Source: CAD feature listing. Evaluate the final solid. Frame: model axes, mm. Round coordinates to 2 decimals unless told otherwise and drop trailing zeros. Use one line per item in the form item = value. Start each with the question number.
Q1. Ray query, line 1 (X direction, y = 5.25, z = 22.5); line 2 (Z direction, x = -54, y = 3.25) (3 decimals). Return the intervals inside material, ascending. Write a range as [from, to].
Q2. Pin query (flat end, axial travel): pin 1 Ø4 at (x, z) = (-88, 31) entering from -Y; pin 2 Ø3 at (x, y) = (169.5, 4.5) entering from +Z (3 decimals). Return the tip coordinate at first contact, or that it passes through.
Q3. Cut plane A-A, the plane z = 34. Give the number of separate pieces and of enclosed holes in the cut face, and give its area (3 significant figures).
from build123d import *

# Parameters (mm, degrees)
SKETCH1_W           = 647.7
SKETCH1_H           = 57.15
BOSS_EXTRUDE1_DEPTH = 6.35
SKETCH3_W           = 24.892
SKETCH3_H           = 12
BOSS_EXTRUDE2_DEPTH = 6.35
SKETCH4_W           = 13.208
SKETCH4_H           = 13.208
CUT_EXTRUDE2_DEPTH  = 327.443679101
SKETCH5_W           = 647.7
SKETCH5_H           = 6.35
CUT_EXTRUDE3_DEPTH  = 31.304


with BuildPart() as part:
    # Sketch1 → Boss-Extrude1 (new body)
    with BuildSketch(Plane(origin=(0, 0, 0), x_dir=(1, 0, 0), z_dir=(0, 1, 0))):
        Rectangle(SKETCH1_W, SKETCH1_H)
    extrude(amount=BOSS_EXTRUDE1_DEPTH)

    # Sketch3 → Boss-Extrude2 (add)
    with BuildSketch(Plane(origin=(0, 0, 0), x_dir=(1, 0, 0), z_dir=(0, 1, 0))):
        Polygon((-317.5, -40.575), (-292.608, -40.575), (-292.608, -28.575), (-317.5, -28.575), (-323.85, -28.575), (-323.85, -40.575), align=None)
        with Locations((-266.954, -34.575)):
            Rectangle(SKETCH3_W, SKETCH3_H)
        with Locations((-228.854, -34.575)):
            Rectangle(SKETCH3_W, SKETCH3_H)
        with Locations((-190.754, -34.575)):
            Rectangle(SKETCH3_W, SKETCH3_H)
        with Locations((-152.654, -34.575)):
            Rectangle(SKETCH3_W, SKETCH3_H)
        with Locations((-114.554, -34.575)):
            Rectangle(SKETCH3_W, SKETCH3_H)
        with Locations((-76.454, -34.575)):
            Rectangle(SKETCH3_W, SKETCH3_H)
        with Locations((-38.354, -34.575)):
            Rectangle(SKETCH3_W, SKETCH3_H)
        with Locations((-0.254, -34.575)):
            Rectangle(SKETCH3_W, SKETCH3_H)
        with Locations((37.846, -34.575)):
            Rectangle(SKETCH3_W, SKETCH3_H)
        with Locations((75.946, -34.575)):
            Rectangle(SKETCH3_W, SKETCH3_H)
        with Locations((114.046, -34.575)):
            Rectangle(SKETCH3_W, SKETCH3_H)
        with Locations((152.146, -34.575)):
            Rectangle(SKETCH3_W, SKETCH3_H)
        with Locations((190.246, -34.575)):
            Rectangle(SKETCH3_W, SKETCH3_H)
        with Locations((228.346, -34.575)):
            Rectangle(SKETCH3_W, SKETCH3_H)
        with Locations((266.446, -34.575)):
            Rectangle(SKETCH3_W, SKETCH3_H)
        Polygon((316.992, -28.575), (292.1, -28.575), (292.1, -40.575), (316.992, -40.575), (323.85, -40.575), (323.85, -28.575), align=None)
    extrude(amount=BOSS_EXTRUDE2_DEPTH)

    # Sketch4 → Cut-Extrude2 (cut, through all)
    with BuildSketch(Plane(origin=(0, 0, 0), x_dir=(1, 0, 0), z_dir=(0, 1, 0))):
        with Locations((-323.85, 3.875)):
            Rectangle(SKETCH4_W, SKETCH4_H)
        with Locations((-323.85, -22.133)):
            Rectangle(SKETCH4_W, SKETCH4_H)
        with Locations((323.85, -22.133)):
            Rectangle(SKETCH4_W, SKETCH4_H)
        with Locations((323.85, 3.875)):
            Rectangle(SKETCH4_W, SKETCH4_H)
        with Locations((-323.85, -48.141)):
            Rectangle(SKETCH4_W, SKETCH4_H)
        with Locations((323.85, -48.141)):
            Rectangle(SKETCH4_W, SKETCH4_H)
    extrude(amount=CUT_EXTRUDE2_DEPTH, mode=Mode.SUBTRACT)

    # Sketch5 → Cut-Extrude3 (cut)
    with BuildSketch(Plane(origin=(0, 0, -28.575), x_dir=(-1, 0, 0), z_dir=(0, 0, -1))):
        with Locations((0, 3.175)):
            Rectangle(SKETCH5_W, SKETCH5_H)
    extrude(amount=-CUT_EXTRUDE3_DEPTH, mode=Mode.SUBTRACT)


solid = part.part
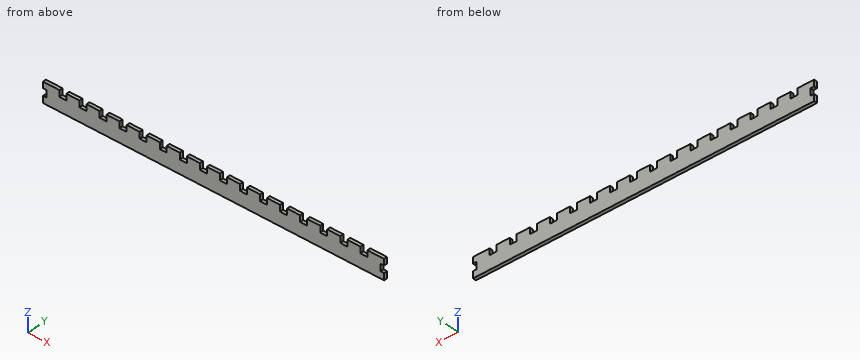
Completed:
q1.line_1 = [-317.25, 317.25]
q1.line_2 = [2.729, 28.575]
q2.pin_1 = 0
q2.pin_2 = 28.575
q3.separate_pieces = 17
q3.enclosed_holes = 0
q3.area = 2,770 mm2
